For this review, take the finished solid that the model builds, in its own axes (mm). Face numbers are marked on the shaded views. Coordinates: 2 decimals unless noted, no trailing zeros. Write each loop counter-clockwise with the first axis right and the second up, starting at its lowest first coordinate (ties: lowest second). Pieces come first, ordered by that corner, then holes. Notation, with made-up numbers: (-5.75, 80.5) -> (9.25, 80.5) arc R21 ccw to (9.25, 106.5) -> close; hole circle Ø7 at (-35, 13). An arc over 180 degrees is marked (long way). Put each result on its own line as item: value. Start each with the question number.
Item 1: Consider section D-D on y = -2. Give the number of separate pieces and of enclosed holes in the cut face, and give its area (3 significant figures).
Item 2: Insertion check: P1, Ø1.5, axis at y = 6, z = -7.5, coming from the +X side; P2, Ø2, axis at x = -4, y = -5.5, coming from the -Z side; P3, Ø4, axis at y = 5, z = 41, coming from the +X side. Each pin has a flat end and moves straight along its axis. Give the tip position at first contact, or say it passes through.
Item 3: Consider section A-A on x = 0. Give the boundary of the cut face in (y, z), and give its area (3 significant figures).
Item 4: To check wall thickness, follow L1, parallel to Z at x = 8.5, y = 3; L2, parallel to Y at x = 0, z = 33; L3, parallel to X at y = -0.75, z = -13. State the ranges of each line that lie inside material, in increasing order.
Item 5: The part is to be moulded in two halves that separate along X. For the marked faces 1, 2, 3 and 4, say which applies: +X half, -X half, draft (parallel to the pull), parting line (faces both ways), or undercut.
Item 6: Consider section B-B on z = 10.5. Give the boundary of the cut face in (x, y).
Item 7: Consider section C-C on z = -4. Give the boundary of the cut face in (x, y).
```python
from build123d import *

# Parameters (mm, degrees)
EXTRUDE1_DEPTH      = 55.794498856
EXTRUDE6_DEPTH      = 9.14463492
EXTRUDE7_REACH      = 59.365
EXTRUDE_THIN1_DEPTH = 9.483751535
SKETCH9_R           = 7.60188161
SKETCH9_R_2         = 6.414649529
EXTRUDE8_DEPTH      = 1.016
SKETCH10_R          = 3.224544811
EXTRUDE9_DEPTH      = 61.86360078
SKETCH2_R           = 7.62
EXTRUDE11_DEPTH     = 55.88
SKETCH12_R          = 9.016750803
EXTRUDE12_DEPTH     = 5.08
SKETCH13_W          = 10.16
SKETCH13_H          = 19.30498436
EXTRUDE13_DEPTH     = 59.71373486
SKETCH16_W          = 10.16
SKETCH16_H          = 10.249002979
EXTRUDE16_DEPTH     = 59.71373486


with BuildPart() as part:
    # Sketch1 → Extrude1 (new body)
    with BuildSketch(Plane.XY):
        with BuildLine():
            Line((-8.715458206, 8.280410535), (8.715458206, 8.280410535))
            Line((8.715458206, 8.280410535), (8.715458206, 0))
            ThreePointArc((8.715458206, 0), (0, -8.715458206), (-8.715458206, 0))
            Line((-8.715458206, 0), (-8.715458206, 8.280410535))
        make_face()
    extrude(amount=EXTRUDE1_DEPTH)

    # Sketch6 → Extrude6 (add, symmetric)
    with BuildSketch(Plane(origin=(0, 0, 0), x_dir=(0, 0, -1), z_dir=(1, 0, 0))):
        with BuildLine():
            Line((0, 8.280410535), (8.988874968, 8.280410535))
            ThreePointArc((8.988874968, 8.280410535), (15.344969413, -7.064558879), (0, -0.708464433))
            Line((0, -0.708464433), (0, 8.280410535))
        make_face()
    extrude(amount=EXTRUDE6_DEPTH, both=True)

    # Sketch7 → Extrude7 (add, up to next)
    with BuildSketch(Plane(origin=(0, 0, 0), x_dir=(-1, 0, 0), z_dir=(0, 0, -1)), mode=Mode.PRIVATE) as extrude7_sk1:
        with BuildLine():
            Line((8.68661556, -0.708464433), (-8.68661556, -0.708464433))
            ThreePointArc((-8.68661556, -0.708464433), (0, -8.715458206), (8.68661556, -0.708464433))
        make_face()
    extrude7_tool1 = extrude(extrude7_sk1.sketch, amount=EXTRUDE7_REACH, mode=Mode.PRIVATE) - part.part
    add(extrude7_tool1.solids().sort_by_distance((0, -4.084646, 0))[0])

    # Sketch8 → Extrude-Thin1 (add, symmetric)
    with BuildSketch(Plane(origin=(0, 0, 0), x_dir=(0, 0, -1), z_dir=(1, 0, 0))):
        with BuildLine():
            ThreePointArc((17.977749936, -0.708464433), (15.344969413, 5.647630012), (8.988874968, 8.280410535))
            Line((8.988874968, 8.280410535), (0, 8.280410535))
            Line((0, 8.280410535), (-57.125499776, 8.280410535))
            Line((-57.125499776, 8.280410535), (-57.125499776, 9.607644959))
            Line((-57.125499776, 9.607644959), (0, 9.607644959))
            Line((0, 9.607644959), (8.988874968, 9.607644959))
            ThreePointArc((8.988874968, 9.607644959), (16.283465875, 6.586126473), (19.30498436, -0.708464433))
            Line((19.30498436, -0.708464433), (17.977749936, -0.708464433))
        make_face()
    extrude(amount=EXTRUDE_THIN1_DEPTH, both=True)

    # Sketch9 → Extrude8 (cut)
    with BuildSketch(Plane(origin=(9.14463492, 0, 0), x_dir=(0, 0, -1), z_dir=(1, 0, 0))):
        with Locations((8.988874968, -0.708464433)):
            Circle(SKETCH9_R)
        with Locations((8.988874968, -0.708464433)):
            Circle(SKETCH9_R_2, mode=Mode.SUBTRACT)
    extrude8 = extrude(amount=-EXTRUDE8_DEPTH, mode=Mode.SUBTRACT)

    # Sketch10 → Extrude9 (cut, through all)
    with BuildSketch(Plane(origin=(9.14463492, 0, 0), x_dir=(0, 0, -1), z_dir=(1, 0, 0))):
        with Locations((8.988874968, -0.708464433)):
            Circle(SKETCH10_R)
    extrude(amount=-EXTRUDE9_DEPTH, mode=Mode.SUBTRACT)

    # Mirror1: Extrude8 across plane
    add(extrude8.mirror(Plane(origin=(0, 0, 0), x_dir=(0, 0, 1), z_dir=(1, 0, 0))), mode=Mode.SUBTRACT)

    # Sketch2 → Extrude11 (cut)
    with BuildSketch(Plane.XY.offset(55.794498856)):
        Circle(SKETCH2_R)
    extrude(amount=-EXTRUDE11_DEPTH, mode=Mode.SUBTRACT)

    # Sketch12 → Extrude12 (cut, symmetric)
    with BuildSketch(Plane(origin=(0, 0, 0), x_dir=(0, 0, -1), z_dir=(1, 0, 0))):
        with Locations((8.988874968, -0.708464433)):
            Circle(SKETCH12_R)
    extrude(amount=EXTRUDE12_DEPTH, both=True, mode=Mode.SUBTRACT)

    # Sketch13 → Extrude13 (cut, through all)
    with BuildSketch(Plane(origin=(0, 0, 0), x_dir=(1, 0, 0), z_dir=(0, 1, 0))):
        with Locations((0, 9.65249218)):
            Rectangle(SKETCH13_W, SKETCH13_H)
    extrude(amount=-EXTRUDE13_DEPTH, mode=Mode.SUBTRACT)

    # Sketch16 → Extrude16 (cut, through all)
    with BuildSketch(Plane(origin=(0, 0, 0), x_dir=(1, 0, 0), z_dir=(0, 1, 0))):
        with Locations((0, 14.15612703)):
            Rectangle(SKETCH16_W, SKETCH16_H)
    extrude(amount=EXTRUDE16_DEPTH, mode=Mode.SUBTRACT)


solid = part.part
```
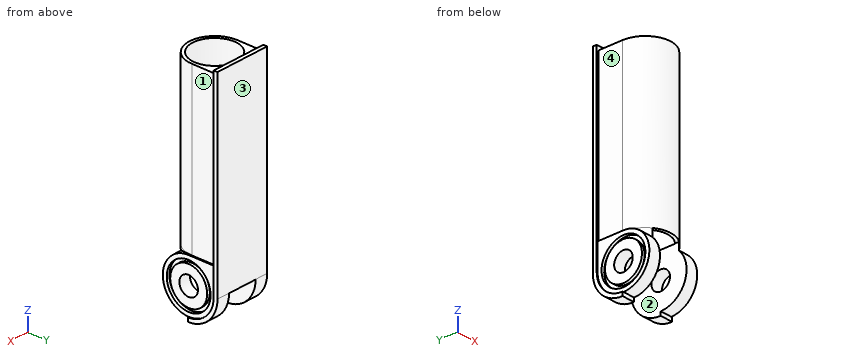
Return value:
1. separate pieces: 4
1. enclosed holes: 0
1. area: 218 mm^2
2. P1: x = 9.14
2. P2: z = 0
2. P3: x = 8.72
3. outline: (-8.72, 0) -> (-7.62, 0) -> (-7.62, 55.79) -> (-8.72, 55.79) -> close; (0.72, -0.09) arc R9.02 cw to (8.31, -9.03) -> (9.61, -9.03) arc R10.32 ccw to (9.61, -8.99) -> (9.61, 57.13) -> (8.28, 57.13) -> (8.28, 55.79) -> (7.62, 55.79) -> (7.62, -0.09) -> close
3. area: 202 mm^2
4. L1: -18.62 to -15.62, -14.22 to -3.75, -2.35 to 55.79
4. L2: -8.72 to -7.62, 7.62 to 9.61
4. L3: -9.14 to -5.08, 5.08 to 9.14
5. face 1: +X half
5. face 2: undercut
5. face 3: draft
5. face 4: -X half
6. outline: (-9.48, 8.28) -> (-8.72, 8.28) -> (-8.72, 0) arc R8.72 ccw to (8.72, 0) -> (8.72, 8.28) -> (9.48, 8.28) -> (9.48, 9.61) -> (-9.48, 9.61) -> close; hole circle Ø15.24 at (0, 0)
7. outline: (-9.48, 8.28) -> (-9.14, 8.28) -> (-9.14, 5.03) -> (-8.13, 5.03) -> (-8.13, 3.32) -> (-9.14, 3.32) -> (-9.14, -4.74) -> (-8.13, -4.74) -> (-8.13, -6.44) -> (-9.14, -6.44) -> (-9.14, -8.19) -> (-5.08, -8.19) -> (-5.08, 6.8) -> (5.08, 6.8) -> (5.08, -8.19) -> (9.14, -8.19) -> (9.14, -6.44) -> (8.13, -6.44) -> (8.13, -4.74) -> (9.14, -4.74) -> (9.14, 3.32) -> (8.13, 3.32) -> (8.13, 5.03) -> (9.14, 5.03) -> (9.14, 8.28) -> (9.48, 8.28) -> (9.48, 9.61) -> (-9.48, 9.61) -> close
